```python
from build123d import *

# Parameters (mm, degrees)
F3_DEPTH        = 34.925
F0_W            = 31.75
F0_H            = 152.4
F7_DEPTH        = 57.15
F7_COPIES_COUNT = 4


# Not quite as in the source:
# - a feature of the source that left no trace in its solid (it failed there, or was rolled back) is left out
# - a pattern or mirror of a feature is missing from the dataset's text; its kind, count and spacing are read off the source's solid


with BuildPart() as f1:
    # F0 (on Front) → F1 (revolve)
    with BuildSketch(Plane.XZ):
        with BuildLine():
            Line((34.925, 73.025), (34.925, 0))
            Line((34.925, 0), (88.9, 0))
            Line((88.9, 0), (88.9, 57.15))
            Line((88.9, 57.15), (63.5, 57.15))
            Line((63.5, 57.15), (63.5, 63.5))
            ThreePointArc((63.5, 63.5), (61.6401280605, 67.9901280605), (57.15, 69.85))
            Line((57.15, 69.85), (54.075, 69.85))
            Line((54.075, 69.85), (54.075, 73.025))
            Line((54.075, 73.025), (34.925, 73.025))
        make_face()
    revolve(axis=Axis((0, 0, -7.5624885379), (0, 0, -1)))

    # F0 (on Front) → F2 (revolve)
    with BuildSketch(Plane.XZ):
        Polygon((0, 1549.4), (0, 0), (34.925, 0), (34.925, 73.025), (34.925, 1549.4), align=None)
    revolve(axis=Axis((0, 0, -7.5624885379), (0, 0, -1)))

    # F0 (on Front) → F3 (join, symmetric)
    with BuildSketch(Plane.XZ):
        Polygon((-34.925, 1549.4), (0, 1549.4), (34.925, 1549.4), (34.925, 1930.4), (31.75, 1930.4), (0, 1930.4), (-34.925, 1930.4), align=None)
    extrude(amount=F3_DEPTH, both=True)

    # F0 (on Front) → F4 (revolve)
    with BuildSketch(Plane.XZ):
        with Locations((15.875, 2006.6)):
            Rectangle(F0_W, F0_H)
    revolve(axis=Axis((0, 0, -7.5624885379), (0, 0, -1)))

    # F6 (on face) → F7 (cut, through all)
    with BuildSketch(Plane(origin=(0, 0, 0), x_dir=(1, 0, 0), z_dir=(0, 0, -1))):
        with BuildLine():
            ThreePointArc((19.05, 60.57513929), (44.9012806053, 44.9012806053), (60.57513929, 19.05))
            Line((60.57513929, 19.05), (86.834944003, 19.05))
            ThreePointArc((86.834944003, 19.05), (62.8617928475, 62.8617928475), (19.05, 86.834944003))
            Line((19.05, 86.834944003), (19.05, 60.57513929))
        make_face()
    f7 = extrude(amount=-F7_DEPTH, mode=Mode.SUBTRACT)

    # F7_copies: F7 ×4 about axis
    f7_copies_axis = Axis((0, 0, 0), (0, 0, 1))
    for i in range(1, F7_COPIES_COUNT):
        add(f7.rotate(f7_copies_axis, i * 360 / F7_COPIES_COUNT), mode=Mode.SUBTRACT)


solid = f1.part
```
For this review, take the finished solid that the model builds, in its own axes (mm). A direction names the side the tool comes from. Round coordinates to 2 decimals unless told otherwise and drop trailing zeros. Order: outer loops, then holes, each group sorted by start corner. A loop starts at its lowest first (then second) coordinate and runs counter-clockwise, first axis right, second up.
Q1. Wall thickness on line 1 (Z direction, x = -33.5, y = 21.5) (3 decimals); line 2 (X direction, y = 4, z = 480); line 3 (Z direction, x = 36.5, y = 4.5) (3 decimals): over which ranges is each line inside the solid? List them lowest first.
Findings below:
line 1: z = 0 to 73.025, 1549.4 to 1930.4
line 2: x = -34.7 to 34.7
line 3: z = 0 to 73.025
Q2. Insertion check: P1, Ø4, axis at x = -30.5, z = 548.5, coming from the -Y side; P2, Ø5, axis at x = -31.5, z = 898, coming from the +Y side; P3, Ø8, axis at y = 17, z = 407.5, coming from the -X side. Each pin has a flat end and moves straight along its axis. Give the tip position at first contact, or say it passes through.
Findings below:
P1: stops at y = -20.19
P2: stops at y = 19.46
P3: stops at x = -32.42
Q3. Mouldability with a two-part tool opening along Z and no side actions: class faces 4 (the flat face through (-28, -27, 1549.4)), 5 (the flat face through (0, 34.925, 1743)), 6 (the flat face through (1, -1, 0)), 7 (the flat face through (-31, -8, 1930.4)) as pulls with the +Z half, pulls with the -Z half, needs draft (parallel to the pull), parting line crosses it, or undercut.
Findings below:
face 4: undercut
face 5: needs draft
face 6: pulls with the -Z half
face 7: pulls with the +Z half
Q4. We need section A-A, the plane z = 1365. Give the boundary of the cut face in (x, y) (3 decimals).
Findings below:
outline: circle Ø69.85 at (0, 0)
Q5. Machinability: for faces 1 (the flat face through (28, 28, 1549.4)), 2 (the flat face through (34.925, 0, 1737)), 3 (the flat face through (-28, 26, 1549.4)), which of the approach directions +Z, -Z, +X, -X, +Y, -Y give a long, thin tool a straight path to every point of the face, cutting with its end or side? Answer none if there is none.
Findings below:
face 1: +X, +Y
face 2: +Z, +X, +Y, -Y
face 3: -X, +Y
